Geometry: final body of the model. Coordinates: model frame, mm. Give positions to 0.01 mm unless a question says otherwise; leave off trailing zeros. Loops run counter-clockwise (first coordinate to the right, second up) from the corner with the lowest first, then second, coordinate; pieces in that order, holes last. Notation, with made-up numbers: M 73.25,1 L 112.25,1 A26 cw 112.25,19 Z; hole C 85.5,63.25 d9. An arc over 180 degrees is marked long. Put each result on its own line as item: value.
```python
from build123d import *

# Parameters (mm, degrees)
CUT_EXTRUDE1_START = 5
CUT_EXTRUDE1_DEPTH = 1


with BuildPart() as part:
    # Sketch1 → Revolve1 (revolve)
    with BuildSketch(Plane.YZ, mode=Mode.PRIVATE) as revolve1_sk:
        with BuildLine():
            Line((0, -5), (1.5, -5))
            Line((1.5, -5), (1.5, 3))
            Line((1.5, 3), (2.75, 3))
            ThreePointArc((2.75, 3), (1.700183814, 4.447127744), (0, 5))
            Line((0, 5), (0, 3))
            Line((0, 3), (0, -5))
        make_face()
    revolve(revolve1_sk.sketch.rotate(Axis((0, 0, 3), (0, 0, 1)), 90), axis=Axis((0, 0, 3), (0, 0, 1)))

    # Sketch2 → Cut-Extrude1 (cut)
    with BuildSketch(Plane(origin=(0, 0, 0), x_dir=(0, 1, 0), z_dir=(0, 0, 1)).offset(CUT_EXTRUDE1_START)):
        Polygon((1.299038106, 0), (0.649519053, 1.125), (-0.649519053, 1.125), (-1.299038106, 0), (-0.649519053, -1.125), (0.649519053, -1.125), align=None)
    extrude(amount=-CUT_EXTRUDE1_DEPTH, mode=Mode.SUBTRACT)


solid = part.part
```
Item 1: Section B-B on x = -0.5. Output: boundary loops of the cut face in (y, z), then the cut area to 3 significant figures.
Output values:
outline: M -2.7,3 L -1.41,3 L -1.41,-5 L 1.41,-5 L 1.41,3 L 2.7,3 A2.85 ccw 1.01,4.77 L 1.01,4 L -1.01,4 L -1.01,4.77 A2.85 ccw Z
area: 28.6 mm²
Item 2: Section D-D on x = -2. Output: boundary loops of the cut face in (y, z), then the cut area to 3 significant figures.
Output values:
outline: M -1.89,3 L 1.89,3 A2.09 ccw Z
area: 3.24 mm²
Item 3: Mould query, pull axis X, two halves, no side actions, for faces 1 (the flat face through (0, 0, 4)), 2 (the flat face through (1.2, 1.2, 3)), 3 (the cylindrical face through (-1.43, -0.45, -0.94)). Classes: pulls with the +X half, pulls with the -X half, needs draft (parallel to the pull), parting line crosses it, or undercut.
Output values:
face 1: undercut
face 2: needs draft
face 3: parting line crosses it
Item 4: Line query: probe 1 along Z at (x, y) = (-1.05, -0.15); probe 2 along X at (y, z) = (0.45, -1); probe 3 along X at (y, z) = (-1, 2.5). Output: solid intervals per line, ascending. Write a range as [from, to].
Output values:
probe 1: [-5, 4]
probe 2: [-1.43, 1.43]
probe 3: [-1.12, 1.12]
Item 5: Section C-C on z = -1.75. Output: boundary loops of the cut face in (x, y).
Output values:
outline: C 0,0 d3
Item 6: Section A-A on y = 0. Output: boundary loops of the cut face in (x, z) (3 decimals).
Output values:
outline: M -2.75,3 L -1.5,3 L -1.5,-5 L 1.5,-5 L 1.5,3 L 2.75,3 A2.891 ccw 1.125,4.772 L 1.125,4 L -1.125,4 L -1.125,4.772 A2.891 ccw Z
Item 7: Pin query (flat end, axial travel): pin 1 Ø1.5 at (y, z) = (1.5, -2) entering from +X; pin 2 Ø2.5 at (x, y) = (0, 0) entering from +Z; pin 3 Ø3 at (x, z) = (2, -0.5) entering from +Y; pin 4 Ø2 at (x, y) = (-2, -2) entering from -Z. Return the tip coordinate at first contact, or that it passes through.
Output values:
pin 1: x = 1.3
pin 2: z = 4.77
pin 3: y = 1.41
pin 4: z = 3
